Input: dimensioned drawing with shaded views. Units: mm. Origin: part minimum x, y, z. A direction names the side the tool comes from. Coordinates: 2 decimals unless noted, no trailing zeros. Order: outer loops, then holes, each group sorted by start corner. A loop starts at its lowest first (then second) coordinate and runs counter-clockwise, first axis right, second up. Notation, with made-up numbers: (6, 3.25) - (59, 3.25) arc R22 cw to (59, 18.25) - close; hole circle Ø4 at (8, -20.75). An arc over 180 degrees is marked (long way). One line per question, with ' | ' between items. Start each with the question number.
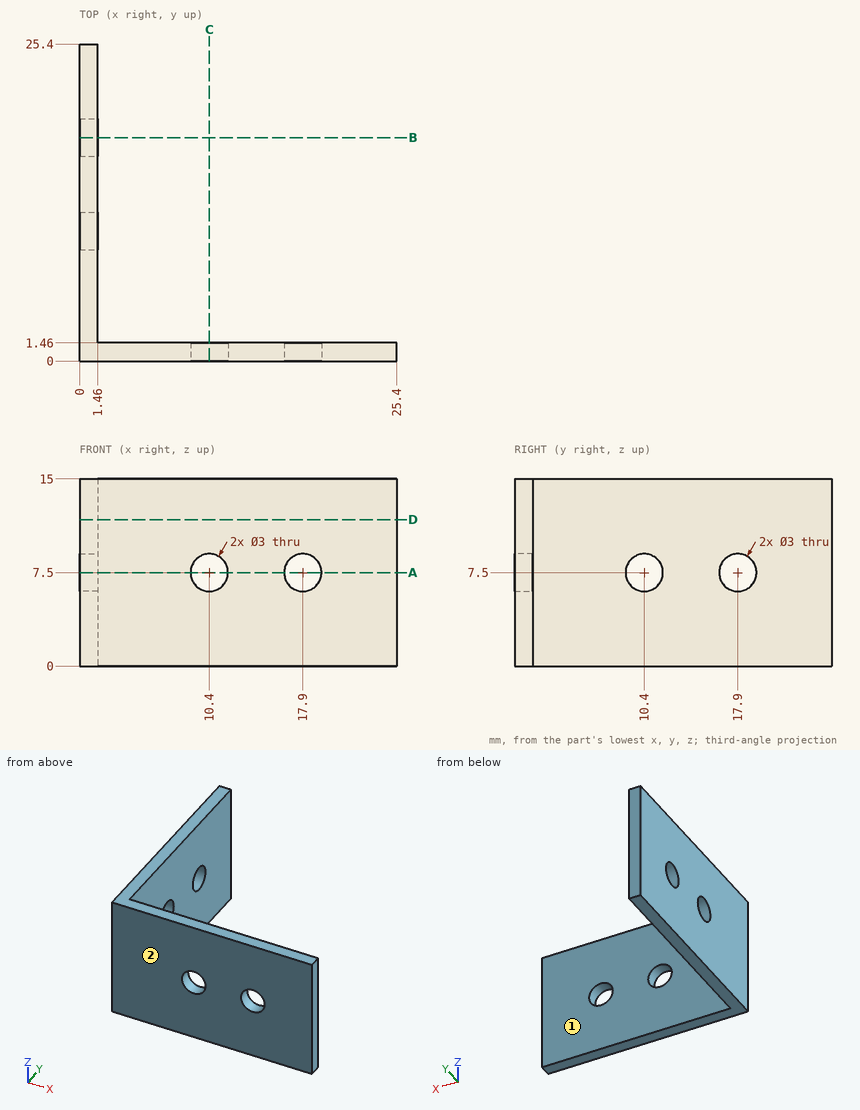
(1) Pin query (flat end, axial travel): pin 1 (5 mm diameter, centred on x = 17.9, z = 7.5, fed in from +Y); pin 2 (2 mm diameter, centred on y = 22, z = 6, fed in from -X); pin 3 (8 mm diameter, centred on y = 7, z = 8, fed in from +X). Return the tip coordinate at first contact, or that it passes through.
(2) Material intervals for line 1 along X through (y, z) = (0.8, 7.5); line 2 along X through (y, z) = (21.5, 7), sorted ascending. Write a range as from..to.
(3) Section B-B (y = 17.9). Output: boundary loops of the cut face in (x, z).
(4) Reachability of the marked faces 1 and 2 from +Z, -Z, +X, -X, +Y, -Y: full face, straight path, thin tool, end or side. Return the list, or none.
(5) Section A-A (z = 7.5). Output: boundary loops of the cut face in (x, y).
(6) Section D-D (z = 11.75). Output: boundary loops of the cut face in (x, y).
Worked answers:
1) pin 1: stops at y = 1.46 | pin 2: stops at x = 0 | pin 3: stops at x = 1.46
2) line 1: x = 0..8.9, 11.9..16.4, 19.4..25.4 | line 2: x = 0..1.46
3) outline: (0, 0) - (1.46, 0) - (1.46, 6) - (0, 6) - close; (0, 9) - (1.46, 9) - (1.46, 15) - (0, 15) - close
4) face 1: +Z, -Z, +X, +Y | face 2: +Z, -Z, +X, -X, -Y
5) outline: (0, 0) - (8.9, 0) - (8.9, 1.46) - (1.46, 1.46) - (1.46, 8.9) - (0, 8.9) - close; (0, 11.9) - (1.46, 11.9) - (1.46, 16.4) - (0, 16.4) - close; (0, 19.4) - (1.46, 19.4) - (1.46, 25.4) - (0, 25.4) - close; (11.9, 0) - (16.4, 0) - (16.4, 1.46) - (11.9, 1.46) - close; (19.4, 0) - (25.4, 0) - (25.4, 1.46) - (19.4, 1.46) - close
6) outline: (0, 0) - (25.4, 0) - (25.4, 1.46) - (1.46, 1.46) - (1.46, 25.4) - (0, 25.4) - close
